```python
from build123d import *

# Parameters (mm, degrees)
F1_DEPTH = 635
F2_R     = 76.2
F2_R_2   = 17.4625
F3_DEPTH = 25.4


with BuildPart() as f1:
    # F0 (on Right) → F1 (new body)
    with BuildSketch(Plane.YZ):
        with BuildLine():
            ThreePointArc((-3.046519, 13.231003), (-7.536648, 11.371131), (-9.396519, 6.881003))
            Line((-9.396519, 6.881003), (-9.396519, -4.605605))
            Line((-9.396519, -4.605605), (9.653481, -4.605605))
            Line((9.653481, -4.605605), (9.653481, 0))
            Line((9.653481, 0), (40.864997, 0))
            Line((40.864997, 0), (40.864997, -4.284248))
            Line((40.864997, -4.284248), (295.403481, -4.284248))
            Line((295.403481, -4.284248), (295.403481, 13.231003))
            Line((295.403481, 13.231003), (-3.046519, 13.231003))
        make_face()
    extrude(amount=F1_DEPTH)

    # F2 (on face) → F3 (cut)
    with BuildSketch(Plane.XY.offset(13.231003)):
        with Locations((114.3, 143.003481)):
            Circle(F2_R)
        with Locations((495.3, 143.003481)):
            Circle(F2_R)
        with Locations((533.4, 238.253481)):
            Circle(F2_R_2)
        with Locations((152.4, 238.253481)):
            Circle(F2_R_2)
    extrude(amount=-F3_DEPTH, mode=Mode.SUBTRACT)


solid = f1.part
```
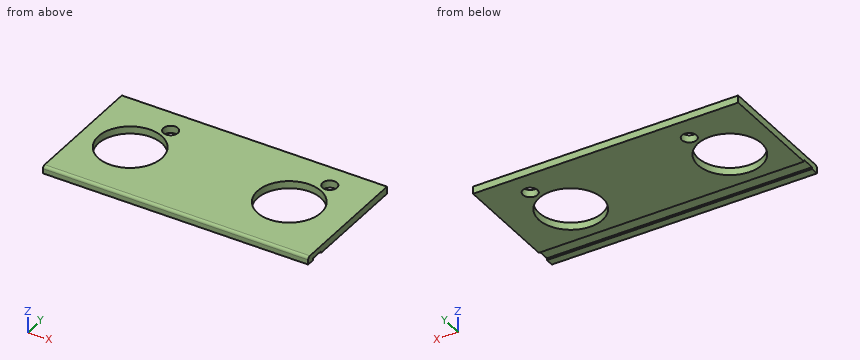
For this review, take the finished solid that the model builds, in its own axes (mm). Round coordinates to 2 decimals unless told otherwise and drop trailing zeros. Write each loop counter-clockwise with the first axis right and the second up, starting at its lowest first coordinate (ties: lowest second). Pieces come first, ordered by that corner, then holes. Notation, with made-up numbers: M 76.25,42.25 L 135.25,42.25 A16 ccw 135.25,62.25 Z; hole C 0,4.25 d6. An arc over 180 degrees is marked long. One line per item, written item: value. Start each with the question number.
(1) We need section D-D (x = 224). Give the boundary of the cut face in (y, z) (3 decimals).
(2) We need section A-A (x = 114.3). Give the boundary of the cut face in (y, z) (3 decimals), and give its area (3 significant figures).
(3) We need section B-B (y = 176). Give the boundary of the cut face in (x, z).
(4) Wall thickness on line 1 (X direction, y = 238, z = 8.5); line 2 (X direction, y = 134, z = 9); line 3 (Y direction, x = 79, z = -1.5) (3 decimals): over which ranges is each line inside the solid? List them lowest first.
(5) Insertion check: pin 1 (12 mm diameter, centred on x = 65, y = 207.5, fed in from -Z); pin 2 (9.5 mm diameter, centred on x = 464.5, y = 21, fed in from -Z). Each pin has a flat end and moves straight along its axis. Give the tip position at first contact, or say it passes through.
(6) We need section C-C (z = 10.5). Give the boundary of the cut face in (x, y) (1 decimal).
Result:
1. outline: M -9.397,-4.606 L 9.653,-4.606 L 9.653,0 L 40.865,0 L 40.865,-4.284 L 295.403,-4.284 L 295.403,13.231 L -3.047,13.231 A6.35 ccw -9.397,6.881 Z
2. outline: M -9.397,-4.606 L 9.653,-4.606 L 9.653,0 L 40.865,0 L 40.865,-4.284 L 66.803,-4.284 L 66.803,13.231 L -3.047,13.231 A6.35 ccw -9.397,6.881 Z; M 219.203,-4.284 L 295.403,-4.284 L 295.403,13.231 L 219.203,13.231 Z
2. area: 2,530 mm²
3. outline: M 0,-4.28 L 45.61,-4.28 L 45.61,13.23 L 0,13.23 Z; M 182.99,-4.28 L 426.61,-4.28 L 426.61,13.23 L 182.99,13.23 Z; M 563.99,-4.28 L 635,-4.28 L 635,13.23 L 563.99,13.23 Z
4. line 1: 0 to 134.94, 169.86 to 515.94, 550.86 to 635
4. line 2: 0 to 38.63, 189.97 to 419.63, 570.97 to 635
4. line 3: -9.397 to 9.653, 40.865 to 75.473, 210.534 to 295.403
5. pin 1: z = -4.28
5. pin 2: z = 0
6. outline: M 0,-8.3 L 635,-8.3 L 635,295.4 L 0,295.4 Z; hole C 114.3,143 d152.4; hole C 152.4,238.3 d34.9; hole C 495.3,143 d152.4; hole C 533.4,238.3 d34.9
